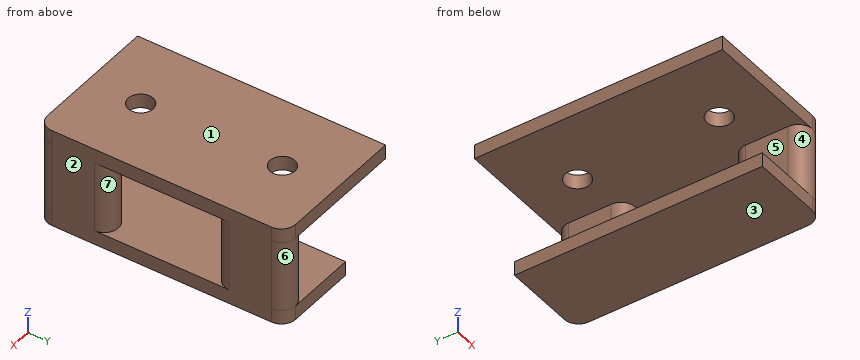
from build123d import *

# Parameters (mm, degrees)
ESQUISSE1_W        = 20
ESQUISSE1_H        = 35
ESQUISSE1_R        = 1.75
BOSS_EXTRU_1_DEPTH = 2
BOSS_EXTRU_2_DEPTH = 10
ESQUISSE3_W        = 12
ESQUISSE3_H        = 35
BOSS_EXTRU_3_DEPTH = 2
CONG_1_R           = 2


with BuildPart() as part:
    # Esquisse1 → Boss.-Extru.1 (new body)
    with BuildSketch(Plane.XY):
        with Locations((-6.602456785, 20.295838232)):
            Rectangle(ESQUISSE1_W, ESQUISSE1_H)
        with Locations((-6.602456785, 30.295838232)):
            Circle(ESQUISSE1_R, mode=Mode.SUBTRACT)
        with Locations((-6.602456785, 10.295838232)):
            Circle(ESQUISSE1_R, mode=Mode.SUBTRACT)
    extrude(amount=-BOSS_EXTRU_1_DEPTH)

    # Esquisse2 → Boss.-Extru.2 (add)
    with BuildSketch(Plane(origin=(0, 0, -2), x_dir=(-1, 0, 0), z_dir=(0, 0, -1))):
        with BuildLine():
            Line((0.602456785, 35.795838232), (0.602456785, 29.795838232))
            ThreePointArc((0.602456785, 29.795838232), (-1.397543215, 27.795838232), (-3.397543215, 29.795838232))
            Line((-3.397543215, 29.795838232), (-3.397543215, 35.795838232))
            ThreePointArc((-3.397543215, 35.795838232), (-1.397543215, 37.795838232), (0.602456785, 35.795838232))
        make_face()
        with BuildLine():
            Line((0.602456785, 4.795838232), (0.602456785, 10.795838232))
            ThreePointArc((0.602456785, 10.795838232), (-1.397543215, 12.795838232), (-3.397543215, 10.795838232))
            Line((-3.397543215, 10.795838232), (-3.397543215, 4.795838232))
            ThreePointArc((-3.397543215, 4.795838232), (-1.397543215, 2.795838232), (0.602456785, 4.795838232))
        make_face()
    extrude(amount=BOSS_EXTRU_2_DEPTH)

    # Esquisse3 → Boss.-Extru.3 (add)
    with BuildSketch(Plane(origin=(0, 0, -12), x_dir=(-1, 0, 0), z_dir=(0, 0, -1))):
        with Locations((2.602456785, 20.295838232)):
            Rectangle(ESQUISSE3_W, ESQUISSE3_H)
    extrude(amount=BOSS_EXTRU_3_DEPTH)

    # Congé1
    cong_1_edges = [part.edges().sort_by_distance(p)[0] for p in [
        (3.397543215, 2.795838232, -1),
        (3.397543215, 37.795838232, -13),
        (3.397543215, 2.795838232, -13),
        (3.397543215, 37.795838232, -1),
    ]]
    fillet(cong_1_edges, radius=CONG_1_R - 0.0001)  # a hair under: the kernel refuses the full size


solid = part.part
Work out the finished part from the listing and answer in its coordinate system (mm). Face numbers are marked on the shaded views. A direction names the side the tool comes from. Give positions to 0.01 mm unless a question says otherwise; leave off trailing zeros. Loops run counter-clockwise (first coordinate to the right, second up) from the corner with the lowest first, then second, coordinate; pieces in that order, holes last. Notation, with made-up numbers: (-24.5, 49) -> (0.5, 49) arc R28 ccw to (0.5, 78) -> close; hole circle Ø5 at (66.5, 55). An arc over 180 degrees is marked (long way). Use a Markdown table: item, result. Add a question column.
1. Section A-A on x = -1.75 is taken. Determine the outline of the cut face in (y, z), and give its area (3 significant figures).
2. Flat-ended cylindrical pins translate along their axes: pin 1 Ø1.8 at (y, z) = (7.5, -8) entering from -X; pin 2 Ø3 at (x, z) = (-0.5, -4.5) entering from +Y; pin 3 Ø2 at (y, z) = (28, -13) entering from -X. Find the tip coordinate at first contact, or state that the pin passes through.
3. Section B-B on y = 22 is taken. Determine the outline of the cut face in (x, z), and give its area (3 significant figures).
4. For the marked faces 5, 6 and 7, determine the directions among +Z, -Z, +X, -X, +Y, -Y from which every point of the face is accessible in a straight line to the end or side of a thin tool.
5. Section C-C on x = -6.75 is taken. Determine the outline of the cut face in (y, z), and give its area (3 significant figures).
6. Find the intervals of material crossed by probe 1 along Z at (x, y) = (-3.25, 32); probe 2 along Y at (x, z) = (1.25, -9.75); probe 3 along X at (y, z) = (32.5, -3.75), in increasing order.
7. Determine the mould class of the marked faces 1, 2, 3 and 4 for opening direction Z: released by +Z, released by -Z, zero draft, split by the parting line, or undercut.
Results below:
| question | item | result |
|---|---|---|
| 1 | outline | (2.8, -14) -> (37.8, -14) -> (37.8, -12) -> (2.8, -12) -> close; (2.8, -2) -> (37.8, -2) -> (37.8, 0) -> (2.8, 0) -> close |
| 1 | area | 140 mm^2 |
| 2 | pin 1 | stops at x = -0.6 |
| 2 | pin 2 | stops at y = 37.76 |
| 2 | pin 3 | stops at x = -8.6 |
| 3 | outline | (-16.6, -2) -> (3.4, -2) -> (3.4, 0) -> (-16.6, 0) -> close; (-8.6, -14) -> (3.4, -14) -> (3.4, -12) -> (-8.6, -12) -> close |
| 3 | area | 64.0 mm^2 |
| 4 | face 5 | -X, +Y, -Y |
| 4 | face 6 | +Y |
| 4 | face 7 | none |
| 5 | outline | (2.8, -14) -> (37.8, -14) -> (37.8, -12) -> (2.8, -12) -> close; (2.8, -2) -> (8.55, -2) -> (8.55, 0) -> (2.8, 0) -> close; (12.04, -2) -> (28.55, -2) -> (28.55, 0) -> (12.04, 0) -> close; (32.04, -2) -> (37.8, -2) -> (37.8, 0) -> (32.04, 0) -> close |
| 5 | area | 126 mm^2 |
| 6 | probe 1 | z = -14 to -12, -2 to 0 |
| 6 | probe 2 | y = 2.8 to 12.79, 27.8 to 37.79 |
| 6 | probe 3 | x = -0.6 to 3.4 |
| 7 | face 1 | released by +Z |
| 7 | face 2 | zero draft |
| 7 | face 3 | released by -Z |
| 7 | face 4 | undercut |
